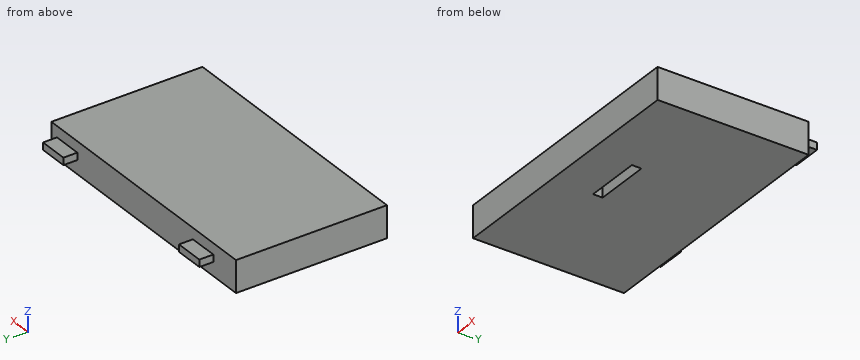
from build123d import *

# Parameters (mm, degrees)
F0_W     = 482.6
F0_H     = 57.8357067246
F1_DEPTH = 275.082
F2_W     = 53.1876
F2_H     = 13.081
F3_DEPTH = 25.4
F5_DEPTH = 25.4


with BuildPart() as f1:
    # F0 (on Front) → F1 (new body)
    with BuildSketch(Plane.XZ):
        with Locations((-28.7254893436, 28.9178533623)):
            Rectangle(F0_W, F0_H)
    extrude(amount=F1_DEPTH)

    # F2 (on face) → F3 (join)
    with BuildSketch(Plane(origin=(0, 0, 0), x_dir=(-1, 0, 0), z_dir=(0, 1, 0))):
        Polygon((-144.7912243771, 37.8729373214), (-197.9788243771, 37.8729373214), (-197.9788243771, 24.7919373214), (-176.1856243771, 24.7919373214), (-144.7912243771, 24.7919373214), align=None)
        with Locations((184.2149756229, 31.3324373214)):
            Rectangle(F2_W, F2_H)
    extrude(amount=F3_DEPTH)

    # F4 (on face) → F5 (cut)
    with BuildSketch(Plane(origin=(0, 0, 0), x_dir=(1, 0, 0), z_dir=(0, 0, -1))):
        Polygon((-63.9737658203, 199.9119593865), (-63.9737658203, 182.5637593865), (37.5036071055, 182.5637593865), (37.6262341797, 199.9119593865), align=None)
    extrude(amount=-F5_DEPTH, mode=Mode.SUBTRACT)


solid = f1.part
Geometry check sheet. Reference: the model listing, model coordinates, mm. Give positions to 0.01 mm unless a question says otherwise; leave off trailing zeros. Write each loop counter-clockwise with the first axis right and the second up, starting at its lowest first coordinate (ties: lowest second). Pieces come first, ordered by that corner, then holes.
1) Cross-section at C-C (x = 3). Record the boundary of the cut face in (y, z), plus the area to 3 significant figures.
Values follow:
outline: (-275.08, 0) - (-199.91, 0) - (-199.91, 25.4) - (-182.56, 25.4) - (-182.56, 0) - (0, 0) - (0, 57.84) - (-275.08, 57.84) - close
area: 15,500 mm2
2) Cross-section at B-B (x = 162). Record the boundary of the cut face in (y, z), plus the area to 3 significant figures.
Values follow:
outline: (-275.08, 0) - (0, 0) - (0, 24.79) - (25.4, 24.79) - (25.4, 37.87) - (0, 37.87) - (0, 57.84) - (-275.08, 57.84) - close
area: 16,200 mm2
3) Cross-section at D-D (x = -236). Record the boundary of the cut face in (y, z), plus the area to 3 significant figures.
Values follow:
outline: (-275.08, 0) - (0, 0) - (0, 57.84) - (-275.08, 57.84) - close
area: 15,900 mm2
4) Thickness scan on line 1 (Y direction, x = -17, z = 3.5); line 2 (X direction, y = -194, z = 18); line 3 (Y direction, x = -134, z = 5.5). Record the ranges inside material, lowest first.
Values follow:
line 1: y = -275.08 to -199.91, -182.56 to 0
line 2: x = -270.03 to -63.97, 37.58 to 212.57
line 3: y = -275.08 to 0
5) Go/stop test with flat-tipped pins: pin 1 Ø6.5 at (y, z) = (14.5, 31.5) entering from -X; pin 2 Ø20.5 at (x, y) = (168, 12) entering from +Z; pin 3 Ø4 at (y, z) = (18, 28.5) entering from +X. Record where each tip stops, or that it passes through.
Values follow:
pin 1: stops at x = -210.81
pin 2: stops at z = 37.87
pin 3: stops at x = 197.98
6) Cross-section at A-A (z = 10). Record the boundary of the cut face in (x, y).
Values follow:
outline: (-270.03, -275.08) - (212.57, -275.08) - (212.57, 0) - (-270.03, 0) - close; hole (-63.97, -199.91) - (37.63, -199.91) - (37.5, -182.56) - (-63.97, -182.56) - close
